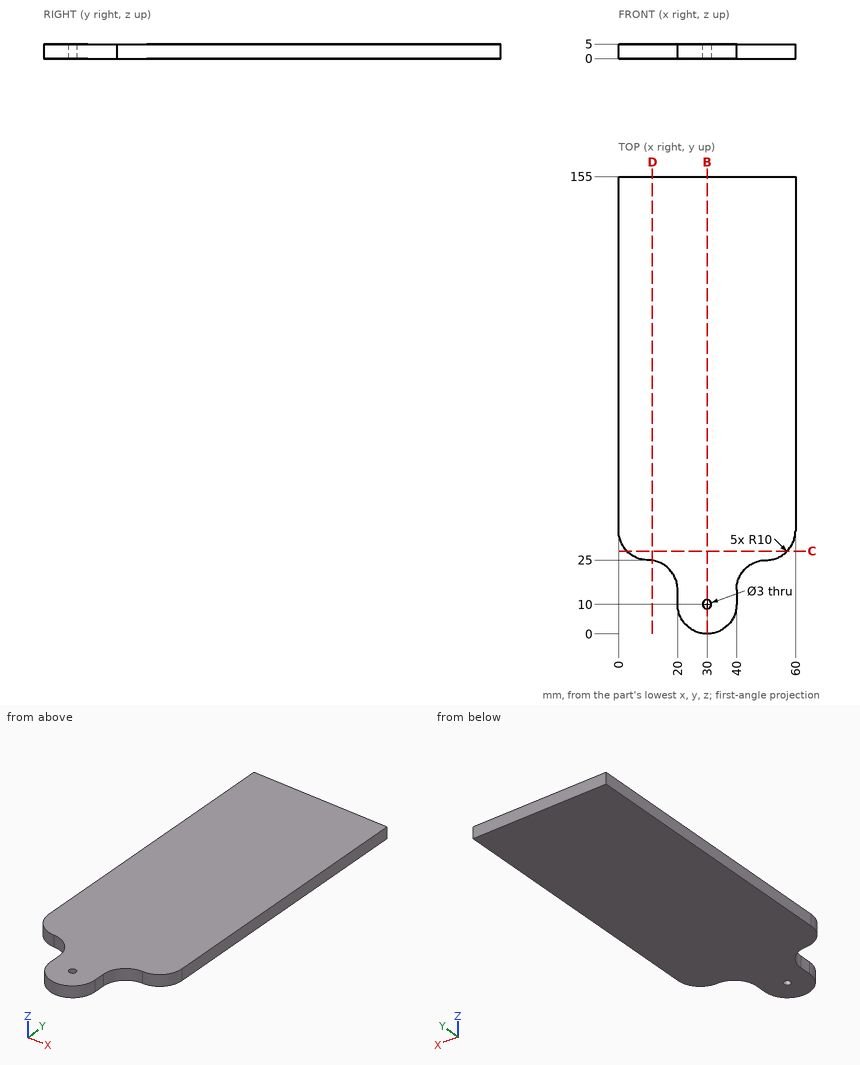
Answer from the drawing. Dimensions are ordinates in mm from the lowest x, y and z of the part. Coordinates: 2 decimals unless noted, no trailing zeros. Write each loop counter-clockwise with the first axis right and the second up, starting at its lowest first coordinate (ties: lowest second). Pieces come first, ordered by that corner, then holes. Notation, with made-up numbers: (49, -5.5) - (59, -5.5) arc R14 ccw to (59, 21.5) - close; hole circle Ø4 at (72.5, -1). An arc over 180 degrees is marked (long way). Return JSON: item names as keys, results as strings. Group by question number.
Q1. The part is cut by section D-D on x = 11.5. Write down the section's boundary in (y, z).
Q2. Flat-ended cylindrical pins translate along their axes: pin 1 Ø2.5 at (y, z) = (12.5, 3.5) entering from -X; pin 2 Ø1.5 at (y, z) = (11.5, 3) entering from +X. Find the tip coordinate at first contact, or state that the pin passes through.
Q3. Find the intervals of material crossed by line 1 along Y through (x, z) = (30, 3.25); line 2 along Y through (x, z) = (45, 2.05); line 3 along Y through (x, z) = (19, 3.7), in increasing order. Write a range as [from, to].
Q4. The part is cut by section C-C on y = 28. Write down the section's boundary in (x, z), and give its area (3 significant figures).
Q5. The part is cut by section B-B on x = 30. Write down the section's boundary in (y, z), and give its area (3 significant figures).
Evaluation:
{
 "1": {"outline": "(24.89, 0) - (155, 0) - (155, 5) - (24.89, 5) - close"},
 "2": {"pin 1": "stops at x = 20", "pin 2": "stops at x = 40"},
 "3": {"line 1": "y = [0, 8.5], [11.5, 155]", "line 2": "y = [23.66, 155]", "line 3": "y = [19.36, 155]"},
 "4": {"outline": "(2.86, 0) - (57.14, 0) - (57.14, 5) - (2.86, 5) - close", "area": "271 mm2"},
 "5": {"outline": "(0, 0) - (8.5, 0) - (8.5, 5) - (0, 5) - close; (11.5, 0) - (155, 0) - (155, 5) - (11.5, 5) - close", "area": "760 mm2"}
}
